Autodesk Inventor part; units mm, degrees
ref_plane "YZ Plane" through (0, 0, 0) normal (1, 0, 0) x (0, 1, 0)
ref_plane "XZ Plane" through (0, 0, 0) normal (0, 1, 0) x (-1, 0, 0)
ref_plane "XY Plane" through (0, 0, 0) normal (0, 0, 1) x (1, 0, 0)
sketch "Sketch1" plane through (0, 0, 0) normal (0, 0, 1) x (1, 0, 0)
  line L0 (-48, 48) -> (48, 48)
  line L1 (48, 48) -> (48, -48)
  line L2 (48, -48) -> (-48, -48)
  line L3 (-48, -48) -> (-48, 48)
  line L4 (38, 38) -> (-38, 38)
  line L5 (-38, 38) -> (-38, -38)
  line L6 (-38, -38) -> (38, -38)
  line L7 (38, -38) -> (38, 38)
  line L8 (0, 152.7233) -> (0, -72.1628) construction
  line L9 (-77.8847, 0) -> (88.8171, 0) construction
  line L10 (-48, 43) -> (48, 43) construction
  line L11 (-43, 48) -> (-43, -48) construction
  line L12 (-48, -43) -> (48, -43) construction
  circle A0 centre (-43, 25) radius 2.25
  circle A1 centre (-43, -25) radius 2.25
  circle A2 centre (-43, -43) radius 2.25
  circle A3 centre (-43, 43) radius 2.25
  line L13 (-48, 30) -> (48, 30) construction
  line L14 (-48, -30) -> (48, -30) construction
  line L15 (-50, 31) -> (-36, 31)
  line L16 (-36, 31) -> (-36, -31)
  line L17 (-36, -31) -> (-50, -31)
  line L18 (-50, -31) -> (-50, 31)
  point P0 (0, 0)
  point P1 (0, 48)
  point P2 (48, 0)
  dimension "d0" = 96
  dimension "d1" = 96
  dimension "d2" = 10
  dimension "d5" = 5
  dimension "d11" = 5
  dimension "d14" = 5
  dimension "d31" = 4.5
  dimension "d32" = 4.5
  dimension "d61" = 4.5
  dimension "d62" = 4.5
  dimension "d65" = 30
  dimension "d66" = 30
  dimension "d67" = 5
  dimension "d68" = 5
  dimension "d74" = 1
  dimension "d75" = 1
  dimension "d76" = 2
  dimension "d77" = 2
extrude "Extrusion1" add sketch "Sketch1" against normal blind 3 contours L0 L1 L2 L3 L17 L5 L6 L7 L4 L15 | L15 L5 L17 L3 | A0 | A1 | A2 | A3
extrude "Extrusion2" cut sketch "Sketch1" against normal blind 10 contours A2 | A3
mirror "Mirror5" about plane through (0, 0, 0) normal (1, 0, 0) of "Extrusion2"
extrude "Extrusion5" cut sketch "Sketch1" against normal blind 10 contours A0 | A1
extrude "Extrusion6" cut sketch "Sketch1" against normal blind 1 contours L15 L5 L17 L3 | L3 L17 L18 L15 | L15 L16 L17 L5
pattern_circular "Circular Pattern1" count 4 over 360 about axis through (0, 0, -10) along (0, 0, 1) of "Extrusion5", "Extrusion6"
equation "\"d31\" = screw"
equation "\"d32\" = screw"
equation "\"d61\" = screw"
equation "\"d62\" = screw"
equation "\"d25\" = mat"
properties part number "Base" material "PC/ABS Plastic"
Part model, mm, in its own coordinate system. A direction names the side the tool comes from. Coordinates: 2 decimals unless noted, no trailing zeros. Order: outer loops, then holes, each group sorted by start corner. A loop starts at its lowest first (then second) coordinate and runs counter-clockwise, first axis right, second up.
(1) Slice it at D-D, the plane y = 43. Write the cut outline in (x, z), and give its area (3 significant figures).
Check sheet entries:
outline: (-48, -3) - (-45.25, -3) - (-45.25, 0) - (-48, 0) - close; (-40.75, -3) - (-27.25, -3) - (-27.25, -1) - (-31, -1) - (-31, 0) - (-40.75, 0) - close; (-22.75, -3) - (22.75, -3) - (22.75, -1) - (-22.75, -1) - close; (27.25, -3) - (40.75, -3) - (40.75, 0) - (31, 0) - (31, -1) - (27.25, -1) - close; (45.25, -3) - (48, -3) - (48, 0) - (45.25, 0) - close
area: 181 mm2
(2) Probe L1, parallel to Y at x = -43, z = -1.7; L2, parallel to Y at x = -15.5, z = -1.9. List the from-to ranges inside material, lowest first.
Check sheet entries:
L1: y = -48 to -45.25, -40.75 to -27.25, -22.75 to 22.75, 27.25 to 40.75, 45.25 to 48
L2: y = -48 to -38, 38 to 48
(3) Slice it at B-B, the plane x = 35. Write the cut outline in (y, z), and give its area (3 significant figures).
Check sheet entries:
outline: (-48, -3) - (-38, -3) - (-38, 0) - (-48, 0) - close; (38, -3) - (48, -3) - (48, 0) - (38, 0) - close
area: 60.0 mm2
(4) Tool access for faces 5 (the face through (-43, 0, -1)), 6 (the face through (-38, 1, -2)), 7 (the face through (0, -43, -1)): list every direction of +Z, -Z, +X, -X, +Y, -Y with a clear straight run to the whole face (end or side of a thin tool).
Check sheet entries:
face 5: +Z, +X, -X
face 6: +Z, -Z
face 7: +Z, +Y, -Y
(5) Slice it at A-A, the plane y = 20.5. Write the cut outline in (x, z).
Check sheet entries:
outline: (-48, -3) - (-38, -3) - (-38, -1) - (-48, -1) - close; (38, -3) - (48, -3) - (48, -1) - (38, -1) - close
(6) Pull direction X, two halves, no side cores. Call faces 1 (the face through (-22.804, -43.488, -1.986)), 2 (the face through (39, -41, 0)), 3 (the face through (48, 1, -2)), 4 (the face through (-1, -38, -2)): pulls with the +X half, pulls with the -X half, needs draft (parallel to the pull), parting line crosses it, or undercut.
Check sheet entries:
face 1: undercut
face 2: needs draft
face 3: pulls with the +X half
face 4: undercut
(7) Pin check, flat tips, straight feed: pin 1 Ø7 at (x, y) = (43, 25) entering from +Z; pin 2 Ø10 at (x, y) = (32.5, 35) entering from -Z. Stop position of each tip, or through.
Check sheet entries:
pin 1: stops at z = -1
pin 2: stops at z = -3
(8) Slice it at C-C, the plane z = -1.7. State how many separate pieces and enclosed holes the cut face has, and give its area (3 significant figures).
Check sheet entries:
separate pieces: 1
enclosed holes: 13
area: 3,250 mm2
